Drawing for the job (mm, zero at the part's lowest x, y, z). A direction names the side the tool comes from. Coordinates: 2 decimals unless noted, no trailing zeros. Order: outer loops, then holes, each group sorted by start corner. A loop starts at its lowest first (then second) coordinate and runs counter-clockwise, first axis right, second up. Notation, with made-up numbers: (9.25, 75) - (27.25, 75) arc R18 cw to (27.25, 108) - close; hole circle Ø7 at (-21.5, 6). An arc over 180 degrees is marked (long way). Answer as CSV lines item,"result". Start each with the question number.
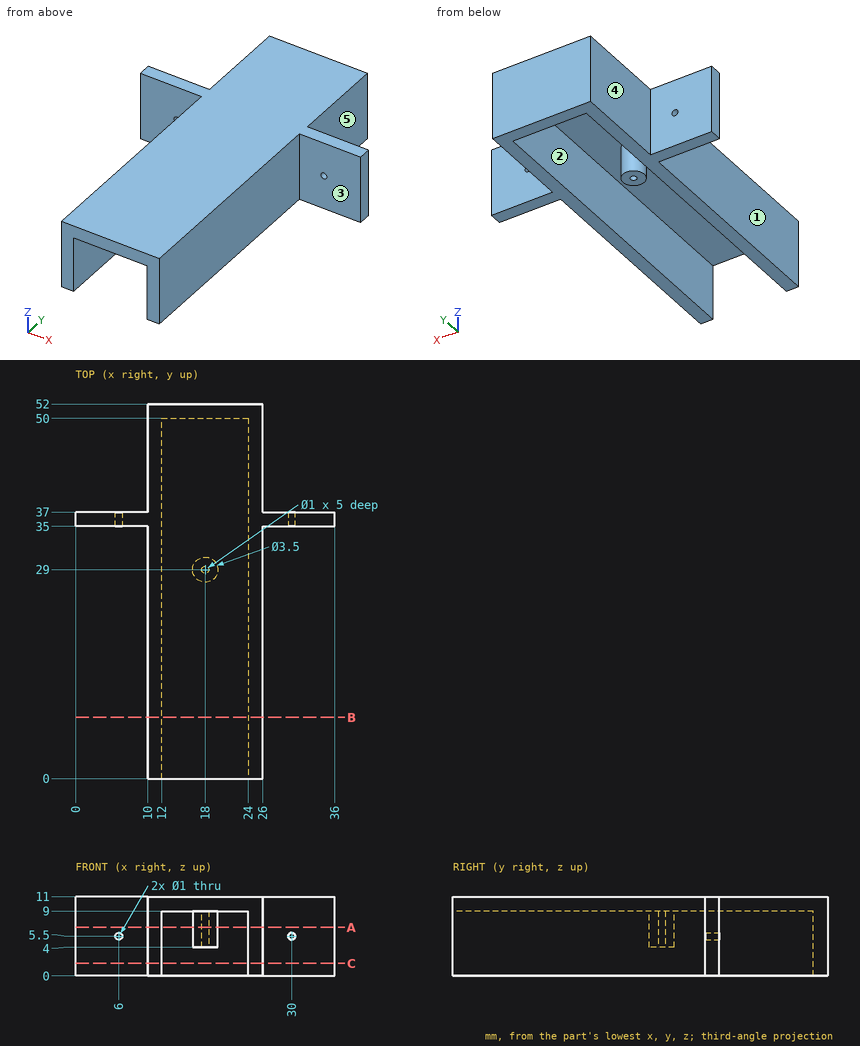
(1) Which spindle directions (+Z, -Z, +X, -X, +Y, -Y) get a long thin tool onto all of the face, cutting with end or side? Do the marked faces 1, 2, 3, 4 and 5. Say none if no direction does.
(2) Band-saw the part on A-A on z = 6.75. List the corners of the cut face in (x, y).
(3) Drop flat-ended pins along their axis: pin 1 Ø0.5 at (x, y) = (18, 29) entering from -Z; pin 2 Ø3 at (y, z) = (27.5, 5) entering from +X; pin 3 Ø5.5 at (y, z) = (9.5, 3.5) entering from -X. Give the stop position or say it passes through.
(4) Band-saw the part on C-C on z = 1.75. List the corners of the cut face in (x, y).
(5) Probe L1, parallel to X at y = 35.55, z = 5.5; L2, parallel to Y at x = 18, z = 5.65; L3, parallel to X at y = 7.5, z = 6.5. List the from-to ranges inside material, lowest first. Write a range as [from, to].
(6) Band-saw the part on B-B on y = 8.5. List the corners of the cut face in (x, z), plus the area to 3 significant figures.
Filled in:
1,face 1,"+Z, -Z, -X, -Y"
1,face 2,"-Z, -Y"
1,face 3,"+Z, -Z, +X, -Y"
1,face 4,"+Z, -Z, -X, +Y"
1,face 5,"+Z, -Z, +X, +Y"
2,outline,"(0, 35) - (10, 35) - (10, 0) - (12, 0) - (12, 50) - (24, 50) - (24, 0) - (26, 0) - (26, 35) - (36, 35) - (36, 37) - (26, 37) - (26, 52) - (10, 52) - (10, 37) - (0, 37) - close; circle Ø3.5 at (18, 29); hole circle Ø1 at (18, 29)"
3,pin 1,"stops at z = 9"
3,pin 2,"stops at x = 26"
3,pin 3,"stops at x = 10"
4,outline,"(0, 35) - (10, 35) - (10, 0) - (12, 0) - (12, 50) - (24, 50) - (24, 0) - (26, 0) - (26, 35) - (36, 35) - (36, 37) - (26, 37) - (26, 52) - (10, 52) - (10, 37) - (0, 37) - close"
5,L1,"x = [0, 5.5], [6.5, 12], [24, 29.5], [30.5, 36]"
5,L2,"y = [27.25, 28.5], [29.5, 30.75], [50, 52]"
5,L3,"x = [10, 12], [24, 26]"
6,outline,"(10, 0) - (12, 0) - (12, 9) - (24, 9) - (24, 0) - (26, 0) - (26, 11) - (10, 11) - close"
6,area,"68.0 mm^2"
